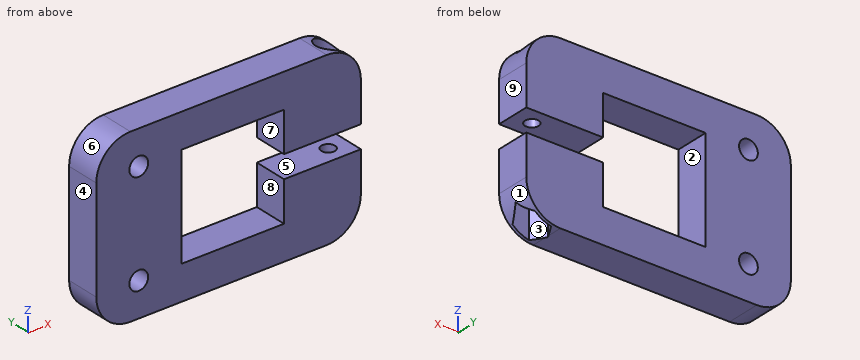
Autodesk Inventor part; units mm, degrees
ref_plane "YZ Plane" through (0, 0, 0) normal (1, 0, 0) x (0, 1, 0)
ref_plane "XZ Plane" through (0, 0, 0) normal (0, 1, 0) x (-1, 0, 0)
ref_plane "XY Plane" through (0, 0, 0) normal (0, 0, 1) x (1, 0, 0)
sketch "Sketch1" plane through (0, 0, 0) normal (0, 1, 0) x (-1, 0, 0)
  line L0 (-15, 15) -> (15, 15)
  line L1 (15, 15) -> (15, -15)
  line L2 (15, -15) -> (-15, -15)
  line L3 (-15, 15) -> (15, -15) construction
  line L4 (15, 15) -> (-15, -15) construction
  line L5 (25, 25) -> (-25, 25)
  line L6 (-25.5008, -25) -> (24.4992, -25)
  line L7 (25, 25) -> (59.45, 25)
  line L8 (59.45, 25) -> (59.45, -25)
  line L9 (59.45, -25) -> (24.4992, -25)
  line L10 (-37.5196, -10.0467) -> (-25.5008, -10.0467)
  line L11 (-25, 10.0467) -> (-37.5196, 10.0467)
  line L12 (-37.5196, -3.2939) -> (-15, -3.2939)
  line L13 (-15, 3.2939) -> (-37.5196, 3.2939)
  line L14 (-37.5196, 10.0467) -> (-37.5196, 3.2939)
  line L15 (-37.5196, -3.2939) -> (-37.5196, -10.0467)
  line L16 (-25, 25) -> (-25, 10.0467)
  line L17 (-15, -15) -> (-15, -3.2939)
  line L18 (-15, 3.2939) -> (-15, 15)
  line L19 (-25.5008, -10.0467) -> (-25.5008, -25)
  point P0 (0, 0)
  point P1 (-30.7833, 0)
  point P2 (25, -25)
  dimension "d0" = 30
  dimension "d1" = 30
  dimension "d2" = 10
  dimension "d4" = 44.45
extrude "Extrusion1" add sketch "Sketch1" along normal blind 10
sketch "Sketch2" plane through (0, 0, 0) normal (0, -1, 0) x (1, 0, 0)
  line L0 (15, 15) -> (-15, 15)
  line L1 (15, 3.2939) -> (15, 15)
  line L2 (37.5196, 3.2939) -> (15, 3.2939)
  line L3 (37.5196, 10.0467) -> (37.5196, 3.2939)
  line L4 (25, 10.0467) -> (37.5196, 10.0467)
  line L5 (25, 25) -> (25, 10.0467)
  line L6 (-59.45, 25) -> (25, 25)
  line L7 (-59.45, -25) -> (-59.45, 25)
  line L8 (25.5008, -25) -> (-59.45, -25)
  line L9 (25.5008, -10.0467) -> (25.5008, -25)
  line L10 (37.5196, -10.0467) -> (25.5008, -10.0467)
  line L11 (37.5196, -3.2939) -> (37.5196, -10.0467)
  line L12 (15, -3.2939) -> (37.5196, -3.2939)
  line L13 (15, -15) -> (15, -3.2939)
  line L14 (-15, -15) -> (15, -15)
  line L15 (-15, 15) -> (-15, -15)
  line L16 (-49.725, -25) -> (-24.725, -25)
  line L17 (-24.725, -25) -> (-24.725, 25)
  line L18 (-24.725, 25) -> (-49.725, 25)
  line L19 (-49.725, 25) -> (-49.725, -25)
  line L20 (-49.725, -25) -> (-24.725, 25) construction
  line L21 (-24.725, -25) -> (-49.725, 25) construction
  line L22 (-59.45, 25) -> (25, 25)
  line L23 (-15, 25) -> (-15, -25)
  line L24 (25.5008, -25) -> (-59.45, -25)
  line L25 (-59.45, 25) -> (-49.725, 25)
  line L26 (-59.45, 25) -> (25, 25)
  line L27 (-24.725, 25) -> (-15, 25)
  line L28 (-59.45, 21.5922) -> (-49.725, 21.5922)
  line L29 (-24.725, 21.5922) -> (-15, 21.5922)
  line L30 (-15, 15) -> (-15, -15)
  point P0 (0, 0)
  point P1 (-37.225, 0)
  point P2 (-15, -25)
  dimension "d7" = 25
extrude "Extrusion2" add sketch "Sketch2" along normal blind 25 contours L15 L23 L8 L17 L29 | L29 L17 L6 L23 | L8 L7 L28 L19 | L19 L28 L7 L6
sketch "Sketch3" plane through (-24.725, 0, -25) normal (-1, 0, 0) x (0, 0, 1)
  line L0 (0, 0) -> (50, 0) construction
  line L1 (0, 0) -> (0, -25) construction
  line L2 (50, -25) -> (0, -25) construction
  line L3 (50, 0) -> (50, -25) construction
  line L4 (0, -12.5) -> (50, -12.5) construction
  line L5 (50, 0) -> (50, -25) construction
  line L6 (15, -12.5) -> (35, -12.5) construction
  line L7 (15, -15.2) -> (35, -15.2) construction
  line L8 (35, -9.8) -> (15, -9.8) construction
  arc A0 (15, -9.8) -> (15, -15.2) centre (15, -12.5) ccw construction
  arc A1 (35, -15.2) -> (35, -9.8) centre (35, -12.5) ccw
  circle A2 centre (35, -12.5) radius 2.7
  circle A3 centre (15, -12.5) radius 2.7
  point P0 (25, 0)
  point P1 (25, -12.5)
  point P2 (35, -9.8)
  dimension "d10" = 20
  dimension "d11" = 2.7
extrude "Extrusion3" cut sketch "Sketch3" along normal through all both and the other way through all
sketch "Sketch4" plane through (37.5196, 0, 10.0467) normal (0, 0, 1) x (1, 0, 0)
  line L0 (-12.5196, 0) -> (0, 0)
  line L1 (0, 0) -> (0, 10)
  line L2 (-12.5196, 10) -> (0, 10)
  circle A0 centre (-5.6081, 5) radius 2
  line L3 (-12.5196, 0) -> (-12.5196, 10)
  point P0 (-37.5196, 0)
  dimension "d15" = 4
extrude "Extrusion4" cut sketch "Sketch4" against normal through all contours A0
sketch "Sketch5" plane through (37.5196, 0, 10.0467) normal (0, 0, 1) x (1, 0, 0)
  circle A0 centre (-5.6081, 5) radius 2
  circle A1 centre (-5.6081, 5) radius 3.6921
  point P0 (-37.5196, 0)
  point P1 (-9.307, 3.7757)
  point P2 (-9.307, 6.2243)
extrude "Extrusion5" cut sketch "Sketch5" along normal mid plane 5 contours A0 | A1
sketch "Sketch6" plane through (0, 10, 0) normal (0, 1, 0) x (1, 0, 0)
  line L0 (25, -25) -> (25, -10.0467)
  line L1 (25, -10.0467) -> (37.5196, -10.0467)
  line L2 (37.5196, -10.0467) -> (37.5196, -3.2939)
  line L3 (37.5196, -3.2939) -> (15, -3.2939)
  line L4 (15, -3.2939) -> (15, -15)
  line L5 (15, -15) -> (-15, -15)
  line L6 (-15, -15) -> (-15, 15)
  line L7 (-15, 15) -> (15, 15)
  line L8 (15, 15) -> (15, 3.2939)
  line L9 (15, 3.2939) -> (37.5196, 3.2939)
  line L10 (37.5196, 3.2939) -> (37.5196, 10.0467)
  line L11 (37.5196, 10.0467) -> (25.5008, 10.0467)
  line L12 (25.5008, 10.0467) -> (25.5008, 25)
  line L13 (25.5008, 25) -> (-59.45, 25)
  line L14 (-59.45, 25) -> (-59.45, -25)
  line L15 (-59.45, -25) -> (25, -25)
  line L16 (-59.45, -25) -> (20, -25)
  line L17 (-25, -25) -> (-25, 25)
  point P0 (0, 0)
  dimension "d20" = 10
  dimension "d21" = 10
extrude "Extrusion6" cut sketch "Sketch6" against normal through all contours L15 L14 L13 L17
sketch "Sketch7" plane through (-24.725, 0, -25) normal (-1, 0, 0) x (0, 0, 1)
  circle A0 centre (35, -12.5) radius 2.7
  circle A1 centre (15, -12.5) radius 2.7
  line L0 (50, -25) -> (0, -25)
  line L1 (50, 0) -> (50, -25)
  line L2 (0, 0) -> (50, 0)
  line L3 (0, 0) -> (0, -25)
  point P0 (25, 0)
extrude "Extrusion7" cut sketch "Sketch7" against normal through all
sketch "Sketch8" plane through (-25, 10, -25) normal (-1, 0, 0) x (0, 0, 1)
  line L0 (50, -10) -> (0, -10)
  line L1 (50, 0) -> (50, -10)
  line L2 (0, 0) -> (50, 0)
  line L3 (0, -10) -> (0, 0)
  point P0 (25, -10)
extrude "Extrusion8" add sketch "Sketch8" along normal blind 15
sketch "Sketch9" plane through (37.5196, 0, -10.0467) normal (0, 0, -1) x (-1, 0, 0)
  circle A0 centre (5.6081, 5) radius 2
  line L0 (0, 0) -> (12.0187, 0)
  line L1 (12.0187, 0) -> (12.0187, 10)
  line L2 (0, 10) -> (12.0187, 10)
  line L3 (0, 0) -> (0, 10)
  circle A1 centre (5.6081, 5) radius 3.6921
  line L4 (7.9753, 9.1) -> (10.3424, 5)
  line L5 (10.3424, 5) -> (7.9753, 0.9)
  line L6 (7.9753, 0.9) -> (3.241, 0.9)
  line L7 (3.241, 0.9) -> (0.8739, 5)
  line L8 (0.8739, 5) -> (3.241, 9.1)
  line L9 (3.241, 9.1) -> (7.9753, 9.1)
  point P0 (37.5196, 0)
  point P1 (8.8062, 2.3392)
  point P2 (8.8062, 7.6608)
  point P3 (8.8062, 6.8449)
  point P4 (8.8062, 3.1551)
  dimension "d28" = 8.2
extrude "Extrusion9" add sketch "Sketch9" along normal up to surface (14.9533 mm away) contours L3 L2 L1 L0
sketch "Sketch10" plane through (25, 0, 10.0467) normal (0, 0, 1) x (1, 0, 0)
  circle A0 centre (6.9114, 5) radius 3.6921
  line L0 (0, 0) -> (12.5196, 0)
  line L1 (12.5196, 0) -> (12.5196, 10)
  line L2 (0, 10) -> (12.5196, 10)
  line L3 (0, 0) -> (0, 10)
  point P0 (-25, 0)
extrude "Extrusion10" add sketch "Sketch10" along normal up to surface (14.9533 mm away)
sketch "Sketch11" plane through (0, 10, 0) normal (0, 1, 0) x (1, 0, 0)
  line L0 (-40.28, -55.2921) -> (-40.28, 159.5519)
  line L1 (-15.12, -75.3901) -> (-15.12, 179.6099)
  line L2 (-40, -25) -> (37.5196, -25)
  line L3 (37.5196, -3.2939) -> (37.5196, -25)
  line L4 (37.5196, -3.2939) -> (15, -3.2939)
  line L5 (15, -3.2939) -> (15, -15)
  line L6 (15, -15) -> (-15, -15)
  line L7 (-15, -15) -> (-15, 15)
  line L8 (-15, 15) -> (15, 15)
  line L9 (15, 15) -> (15, 3.2939)
  line L10 (15, 3.2939) -> (37.5196, 3.2939)
  line L11 (37.5196, 3.2939) -> (37.5196, 25)
  line L12 (37.5196, 25) -> (-40, 25)
  line L13 (-40, -25) -> (-40, 25)
  line L14 (-15.12, 25) -> (-40, 25) construction
  circle A0 centre (-27.56, 15) radius 2.75
  circle A1 centre (-27.56, -15) radius 2.75
  point P0 (0, 0)
  dimension "d33" = 5.5
extrude "Extrusion11" cut sketch "Sketch11" against normal through all contours A0 | A1
fillet "Fillet2" radius 10 4 edges at (37.5196, 5, 25) (37.5196, 5, -25) (-40, 5, 25) (-40, 5, -25)
properties part number "estopMountV2"
Input: part model. Units: mm. Frame: model coordinates. Face numbers are marked on the shaded views. A direction names the side the tool comes from. Coordinates: 2 decimals unless noted, no trailing zeros. Order: outer loops, then holes, each group sorted by start corner. A loop starts at its lowest first (then second) coordinate and runs counter-clockwise, first axis right, second up. Notation, with made-up numbers: (73.25, 31.25) - (97.25, 31.25) arc R29 cw to (97.25, 69.25) - close; hole circle Ø4 at (19.25, -31). An arc over 180 degrees is marked (long way). Put each result on its own line as item: value.
1. Reachability of the marked faces 1, 2, 3, 4 and 5 from +Z, -Z, +X, -X, +Y, -Y: full face, straight path, thin tool, end or side. Return the list, or none.
Report:
face 1: -Z, +X, +Y, -Y
face 2: +Y, -Y
face 3: -Z
face 4: +Z, -Z, -X, +Y, -Y
face 5: +X, +Y, -Y
2. Cut plane C-C on x = -27.56. Return the cut outline in (y, z).
Report:
outline: (0, -25) - (10, -25) - (10, -17.75) - (0, -17.75) - close; (0, -12.25) - (10, -12.25) - (10, 12.25) - (0, 12.25) - close; (0, 17.75) - (10, 17.75) - (10, 25) - (0, 25) - close
3. Cut plane B-B on x = -1.5. Return the cut outline in (y, z).
Report:
outline: (0, -25) - (10, -25) - (10, -15) - (0, -15) - close; (0, 15) - (10, 15) - (10, 25) - (0, 25) - close
4. Cut plane D-D on z = 11. Return the cut outline in (x, y).
Report:
outline: (-40, 0) - (-15, 0) - (-15, 10) - (-40, 10) - close; (15, 0) - (37.52, 0) - (37.52, 10) - (15, 10) - close; hole circle Ø7.38 at (31.91, 5)
5. Cut plane A-A on z = -11.5. Return the cut outline in (x, y), then the cut area to 3 significant figures.
Report:
outline: (-40, 0) - (-15, 0) - (-15, 10) - (-40, 10) - close; (15, 0) - (37.52, 0) - (37.52, 10) - (15, 10) - close; hole (27.18, 5) - (29.54, 0.9) - (34.28, 0.9) - (36.65, 5) - (34.28, 9.1) - (29.54, 9.1) - close
area: 417 mm2
6. Draft query along Z for the marked faces 6, 7, 8 and 9. Return one class per face: pulls with the +Z half, pulls with the -Z half, needs draft (parallel to the pull), parting line crosses it, or undercut.
Report:
face 6: pulls with the +Z half
face 7: undercut
face 8: undercut
face 9: needs draft
7. Contact query for flat-ended pins moving along their axis: pin 1 Ø3.5 at (x, y) = (33, 5.5) entering from +Z; pin 2 Ø2.5 at (x, y) = (34, 4) entering from -Z; pin 3 Ø10 at (x, z) = (-11.5, 8.5) entering from +Y; pin 4 Ø3 at (x, y) = (31.91, 5) entering from -Z. Output: stop coordinate, or through.
Report:
pin 1: stops at z = 7.55
pin 2: stops at z = -10.05
pin 3: stops at y = 10
pin 4: passes through
8. Line query: line 1 along Z through (x, y) = (-27.56, 5.5); line 2 along Z through (x, y) = (-8.5, 7.75); line 3 along Z through (x, y) = (31, 2.75). Output: solid intervals per line, ascending.
Report:
line 1: z = -25 to -17.75, -12.25 to 12.25, 17.75 to 25
line 2: z = -25 to -15, 15 to 25
line 3: z = -10.05 to -3.29, 3.29 to 7.55
